Model file for the job. Use its own axes, mm. A direction names the side the tool comes from. Coordinates: 2 decimals unless noted, no trailing zeros. Write each loop counter-clockwise with the first axis right and the second up, starting at its lowest first coordinate (ties: lowest second). Pieces come first, ordered by that corner, then holes. Notation, with made-up numbers: M -16,48 L 20,48 A20 ccw 20,77 Z; hole C -3.75,88.25 d3. An arc over 180 degrees is marked long. One line per question, with ' | ' between items. Start each with the question number.
(1) Cut at C-C (z = 62). Write the cut outline in (x, y), plus the area to 3 significant figures.
(2) Two-plate mould, pull along Y, no slides. Class faces 1 (the face through (9.098, 0.986, 52.672)), 2 (the face through (16, 10, 51)), 3 (the face through (13, 0, 40)): +Y half, -Y half, draft (parallel to the pull), parting line (faces both ways), or undercut.
(3) Tool access for faces 4 (the face through (18, 17, 95)), 5 (the face through (13, 20, 40)), 6 (the face through (12, 18, 31)): list every direction of +Z, -Z, +X, -X, +Y, -Y with a clear straight run to the whole face (end or side of a thin tool).
(4) Cut at A-A (y = 10). Write the cut outline in (x, z), plus the area to 3 significant figures.
(5) Wall check: probe 1 along Z at (x, y) = (16.75, 3.25); probe 2 along Y at (x, z) = (13, 71); probe 3 along Y at (x, z) = (17.5, 28). Give the ranges that are in metal, low to high.
(6) Flat gauge pins, fed straight in: pin 1 Ø3 at (y, z) = (7.5, 26.5) entering from -X; pin 2 Ø4 at (y, z) = (17, 19) entering from -X; pin 3 Ø5 at (x, y) = (10, 10) entering from +Z. Where does each tip first touch, or does it go through?
(7) Cut at B-B (x = 18). Write the cut outline in (y, z), plus the area to 3 significant figures.
(8) Cut at D-D (x = 10). Write the cut outline in (y, z), plus the area to 3 significant figures.
from build123d import *

# Parameters (mm, degrees)
F0_W      = 20
F0_H      = 20
F0_R      = 2.15
F1_DEPTH  = 4
F2_W      = 4
F2_H      = 20
F3_DEPTH  = 96
F4_W      = 1.5
F4_H      = 6
F5_DEPTH  = 20.001
F6_R      = 2
F8_DEPTH  = 2
F10_DEPTH = 2


with BuildPart() as f1:
    # F0 (on Top) → F1 (new body)
    with BuildSketch(Plane.XY):
        with Locations((10, 10)):
            Rectangle(F0_W, F0_H)
        with Locations((10, 10)):
            Circle(F0_R, mode=Mode.SUBTRACT)
    extrude(amount=F1_DEPTH)

    # F2 (on face) → F3 (join)
    with BuildSketch(Plane.XY.offset(4)):
        with Locations((18, 10)):
            Rectangle(F2_W, F2_H)
    extrude(amount=F3_DEPTH)

    # F4 (on face) → F5 (cut, through all)
    with BuildSketch(Plane.YZ.offset(20)):
        with Locations((3.75, 95)):
            Rectangle(F4_W, F4_H)
        with Locations((16.25, 95)):
            Rectangle(F4_W, F4_H)
        with Locations((3.75, 61.666667)):
            Rectangle(F4_W, F4_H)
        with Locations((16.25, 61.666667)):
            Rectangle(F4_W, F4_H)
        with Locations((3.75, 28.333333)):
            Rectangle(F4_W, F4_H)
        with Locations((16.25, 28.333333)):
            Rectangle(F4_W, F4_H)
    extrude(amount=-F5_DEPTH, mode=Mode.SUBTRACT)

    # F6
    f6_edges = [f1.edges().sort_by_distance(p)[0] for p in [
        (0, 0, 2),
        (0, 20, 2),
    ]]
    fillet(f6_edges, radius=F6_R)

    # F7 (on face) → F8 (join)
    with BuildSketch(Plane.XZ):
        Polygon((16, 4), (16, 100), (2, 4), align=None)
    extrude(amount=-F8_DEPTH)

    # F9 (on face) → F10 (join)
    with BuildSketch(Plane(origin=(0, 20, 0), x_dir=(-1, 0, 0), z_dir=(0, 1, 0))):
        Polygon((-16, 4), (-2, 4), (-16, 100), align=None)
    extrude(amount=-F10_DEPTH)


solid = f1.part
Filled in:
1) outline: M 10.46,0 L 20,0 L 20,3 L 16,3 L 16,2 L 10.46,2 Z; M 10.46,18 L 16,18 L 16,17 L 20,17 L 20,20 L 10.46,20 Z; M 16,4.5 L 20,4.5 L 20,15.5 L 16,15.5 Z | area: 90.2 mm²
2) face 1: draft | face 2: undercut | face 3: -Y half
3) face 4: +X, -X | face 5: +Z, -Z, +X, -X, +Y | face 6: +Z, -X
4) outline: M 0,0 L 7.85,0 L 7.85,4 L 0,4 Z; M 12.15,0 L 20,0 L 20,100 L 16,100 L 16,4 L 12.15,4 Z | area: 447 mm²
5) probe 1: 0 to 25.33, 31.33 to 58.67, 64.67 to 92, 98 to 100 | probe 2: 0 to 2, 18 to 20 | probe 3: 0 to 3, 4.5 to 15.5, 17 to 20
6) pin 1: x = 16 | pin 2: x = 3.93 | pin 3: z = 4
7) outline: M 0,0 L 20,0 L 20,100 L 0,100 Z; hole M 3,25.33 L 4.5,25.33 L 4.5,31.33 L 3,31.33 Z; hole M 3,58.67 L 4.5,58.67 L 4.5,64.67 L 3,64.67 Z; hole M 3,92 L 4.5,92 L 4.5,98 L 3,98 Z; hole M 15.5,25.33 L 17,25.33 L 17,31.33 L 15.5,31.33 Z; hole M 15.5,58.67 L 17,58.67 L 17,64.67 L 15.5,64.67 Z; hole M 15.5,92 L 17,92 L 17,98 L 15.5,98 Z | area: 1,950 mm²
8) outline: M 0,0 L 7.85,0 L 7.85,4 L 2,4 L 2,58.86 L 0,58.86 Z; M 12.15,0 L 20,0 L 20,58.86 L 18,58.86 L 18,4 L 12.15,4 Z | area: 282 mm²
